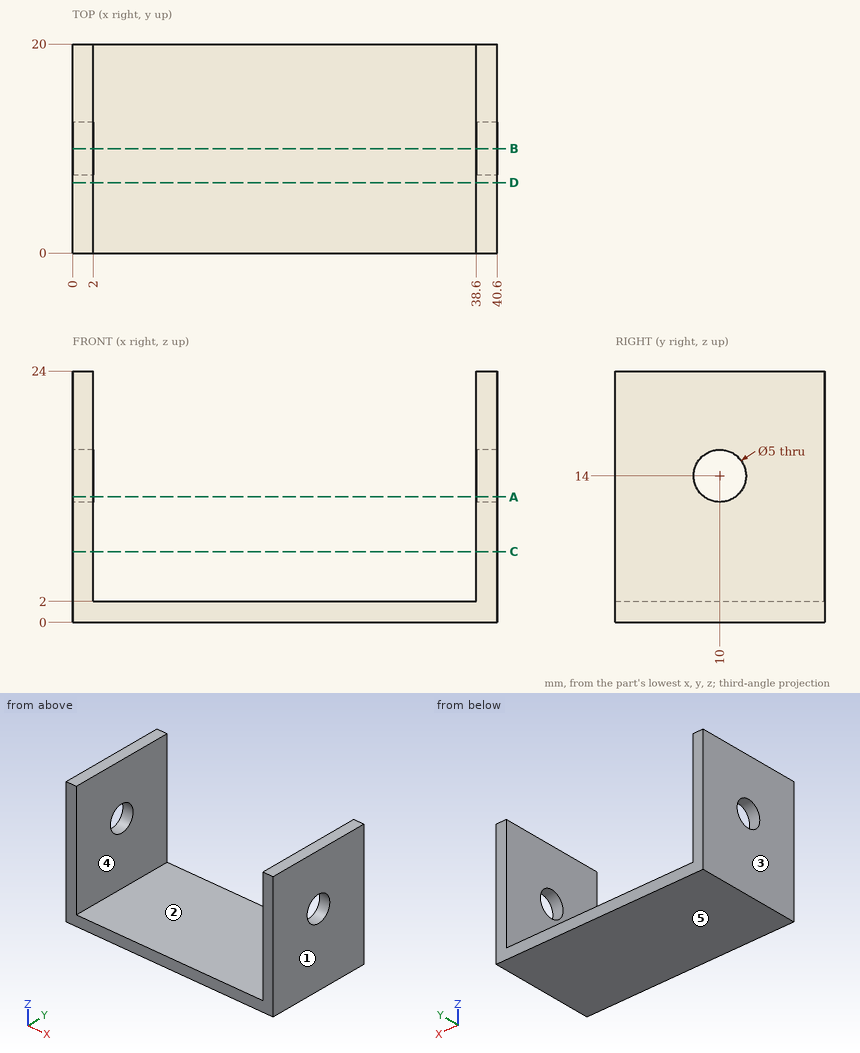
For this review, use the dimensioned drawing (mm, ordinates from the lowest corner) and the shaded views. A direction names the side the tool comes from. Coordinates: 2 decimals unless noted, no trailing zeros. Write each loop counter-clockwise with the first axis right and the second up, starting at its lowest first coordinate (ties: lowest second). Pieces come first, ordered by that corner, then holes. Notation, with made-up numbers: (85.5, -34) - (103.5, -34) arc R10 cw to (103.5, -17) - close; hole circle Ø2 at (70, 21). An arc over 180 degrees is marked (long way). One line per item, written item: value.
1) Insertion check: pin 1 (6 mm diameter, centred on y = 4.5, z = 4.5, fed in from -X); pin 2 (6 mm diameter, centred on x = 19, y = 5, fed in from +Z); pin 3 (4 mm diameter, centred on x = 32, z = 4.5, fed in from -Y). Each pin has a flat end and moves straight along its axis. Give the tip position at first contact, or say it passes through.
Answer sheet:
pin 1: stops at x = 0
pin 2: stops at z = 2
pin 3: passes through
2) To check wall thickness, follow probe 1 along Z at (x, y) = (0.8, 10); probe 2 along X at (y, z) = (11, 7.25); probe 3 along Z at (x, y) = (13, 2.25). State the ranges of each line that lie inside material, in increasing order.
Answer sheet:
probe 1: z = 0 to 11.5, 16.5 to 24
probe 2: x = 0 to 2, 38.6 to 40.6
probe 3: z = 0 to 2
3) Add section D-D (y = 6.75). State the section outline as (x, z) points.
Answer sheet:
outline: (0, 0) - (40.6, 0) - (40.6, 24) - (38.6, 24) - (38.6, 2) - (2, 2) - (2, 24) - (0, 24) - close
4) Mouldability with a two-part tool opening along X and no side actions: class the marked faces 3, 4 and 5 as +X half, -X half, draft (parallel to the pull), parting line (faces both ways), or undercut.
Answer sheet:
face 3: -X half
face 4: undercut
face 5: draft
5) Add section B-B (y = 10). State the section outline as (x, z) points.
Answer sheet:
outline: (0, 0) - (40.6, 0) - (40.6, 11.5) - (38.6, 11.5) - (38.6, 2) - (2, 2) - (2, 11.5) - (0, 11.5) - close; (0, 16.5) - (2, 16.5) - (2, 24) - (0, 24) - close; (38.6, 16.5) - (40.6, 16.5) - (40.6, 24) - (38.6, 24) - close
6) For the marked faces 1 and 2, list the 3-axis set-ups (+Z, -Z, +X, -X, +Y, -Y) from which the entire face can be reached by the end or side of a thin tool; tool diameter is ignored.
Answer sheet:
face 1: +Z, -Z, +X, +Y, -Y
face 2: +Z, +Y, -Y
7) Add section C-C (z = 6.75). State the section outline as (x, y) points.
Answer sheet:
outline: (0, 0) - (2, 0) - (2, 20) - (0, 20) - close; (38.6, 0) - (40.6, 0) - (40.6, 20) - (38.6, 20) - close
8) Add section A-A (z = 12). State the section outline as (x, y) points.
Answer sheet:
outline: (0, 0) - (2, 0) - (2, 8.5) - (0, 8.5) - close; (0, 11.5) - (2, 11.5) - (2, 20) - (0, 20) - close; (38.6, 0) - (40.6, 0) - (40.6, 8.5) - (38.6, 8.5) - close; (38.6, 11.5) - (40.6, 11.5) - (40.6, 20) - (38.6, 20) - close
